Part model, mm, in its own coordinate system. Round coordinates to 2 decimals unless told otherwise and drop trailing zeros. Write each loop counter-clockwise with the first axis right and the second up, starting at its lowest first coordinate (ties: lowest second). Pieces come first, ordered by that corner, then holes. Notation, with made-up numbers: M 63.5,83.5 L 69.5,83.5 A26 ccw 69.5,116.5 Z; hole C 74.25,43.5 d1. An arc over 180 degrees is marked long. One line per question, with ' | ' between items. Start each with the question number.
1) Saw through at B-B (z = -19). List the corners of the cut face in (x, y), plus the area to 3 significant figures.
2) Saw through at A-A (x = 23). List the corners of the cut face in (y, z) (3 decimals).
3) Saw through at C-C (y = 20.5). List the corners of the cut face in (x, z), plus the area to 3 significant figures.
4) Wall check: probe 1 along Y at (x, z) = (30.5, -21); probe 2 along Y at (x, z) = (32, -37); probe 3 along Z at (x, y) = (26, 18). Give the ranges that are in metal, low to high. Write a range as [from, to].
```python
from build123d import *

# Parameters (mm, degrees)
SKETCH1_W           = 42.418
SKETCH1_H           = 46.99
BOSS_EXTRUDE1_DEPTH = 32.258
CUT_EXTRUDE1_DEPTH  = 43.418


with BuildPart() as part:
    # Sketch1 → Boss-Extrude1 (new body)
    with BuildSketch(Plane(origin=(0, 0, 0), x_dir=(1, 0, 0), z_dir=(0, 1, 0))):
        with Locations((21.209, 23.495)):
            Rectangle(SKETCH1_W, SKETCH1_H)
    extrude(amount=BOSS_EXTRUDE1_DEPTH)

    # Sketch2 → Cut-Extrude1 (cut, through all)
    with BuildSketch(Plane(origin=(42.418, 0, 0), x_dir=(0, 0, -1), z_dir=(1, 0, 0))):
        with BuildLine():
            Line((10.495, 22.054113), (36.495, 22.054113))
            ThreePointArc((36.495, 22.054113), (38.991113, 19.558), (36.495, 17.061887))
            Line((36.495, 17.061887), (10.495, 17.061887))
            ThreePointArc((10.495, 17.061887), (7.998887, 19.558), (10.495, 22.054113))
        make_face()
    extrude(amount=-CUT_EXTRUDE1_DEPTH, mode=Mode.SUBTRACT)


solid = part.part
```
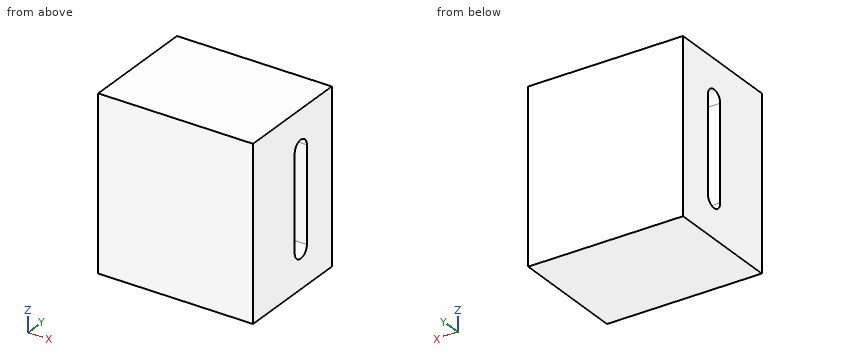
Answer key:
1) outline: M 0,0 L 42.42,0 L 42.42,17.06 L 0,17.06 Z; M 0,22.05 L 42.42,22.05 L 42.42,32.26 L 0,32.26 Z | area: 1,160 mm2
2) outline: M 0,-46.99 L 32.258,-46.99 L 32.258,0 L 0,0 Z; hole M 17.062,-36.495 A2.496 ccw 22.054,-36.495 L 22.054,-10.495 A2.496 ccw 17.062,-10.495 Z
3) outline: M 0,-46.99 L 42.42,-46.99 L 42.42,-38.81 L 0,-38.81 Z; M 0,-8.18 L 42.42,-8.18 L 42.42,0 L 0,0 Z | area: 694 mm2
4) probe 1: y = [0, 17.06], [22.05, 32.26] | probe 2: y = [0, 17.11], [22, 32.26] | probe 3: z = [-46.99, -38.45], [-8.54, 0]
